```python
from build123d import *

# Parameters (mm, degrees)
BOSS_EXTRUDE1_DEPTH              = 20
CUT_EXTRUDE1_DEPTH               = 80
M14X2_0_TAPPED_HOLE2_D           = 12
M14X2_0_TAPPED_HOLE2_CSINK_D     = 14.05
M14X2_0_TAPPED_HOLE2_CSINK_ANGLE = 90
SKETCH11_W                       = 26
SKETCH11_H                       = 50
BOSS_EXTRUDE2_DEPTH              = 60
BOSS_EXTRUDE3_START              = 4
SKETCH12_R                       = 24.50968872
BOSS_EXTRUDE3_DEPTH              = 34
BOSS_EXTRUDE4_START              = 4
SKETCH13_R                       = 24.725624797
BOSS_EXTRUDE4_DEPTH              = 34
SKETCH14_R                       = 10
CUT_EXTRUDE2_DEPTH               = 234
SKETCH15_W                       = 34
SKETCH15_H                       = 100.230824912
CUT_EXTRUDE3_DEPTH               = 6
RIB6_REACH                       = 189.964
SKETCH16_WALL_W                  = 418.569099694
SKETCH16_WALL_H                  = 16


with BuildPart() as part:
    # Sketch1 → Boss-Extrude1 (new body)
    with BuildSketch(Plane.XY):
        with BuildLine():
            Line((-165.913043478, -4.304347826), (54.086956522, -4.304347826))
            ThreePointArc((54.086956522, -4.304347826), (79.086956522, 20.695652174), (54.086956522, 45.695652174))
            Line((54.086956522, 45.695652174), (-165.913043478, 45.695652174))
            Line((-165.913043478, 45.695652174), (-165.913043478, 28.695652174))
            Line((-165.913043478, 28.695652174), (-149.913043478, 28.695652174))
            ThreePointArc((-149.913043478, 28.695652174), (-141.913043478, 20.695652174), (-149.913043478, 12.695652174))
            Line((-149.913043478, 12.695652174), (-165.913043478, 12.695652174))
            Line((-165.913043478, 12.695652174), (-165.913043478, -4.304347826))
        make_face()
    extrude(amount=BOSS_EXTRUDE1_DEPTH)

    # Sketch2 → Cut-Extrude1 (cut)
    with BuildSketch(Plane(origin=(0, 45.695652174, 0), x_dir=(1, 0, 0), z_dir=(0, 1, 0))):
        with BuildLine():
            Line((-80.413043478, -20), (-6.413043478, -20))
            Line((-6.413043478, -20), (-6.413043478, -18))
            ThreePointArc((-6.413043478, -18), (-7.584616354, -15.171572875), (-10.413043478, -14))
            Line((-10.413043478, -14), (-76.413043478, -14))
            ThreePointArc((-76.413043478, -14), (-79.241470603, -15.171572875), (-80.413043478, -18))
            Line((-80.413043478, -18), (-80.413043478, -20))
        make_face()
    extrude(amount=-CUT_EXTRUDE1_DEPTH, mode=Mode.SUBTRACT)

    # M14x2.0 Tapped Hole2 (through all)
    with Locations(Plane(origin=(0, 0, 0), x_dir=(-1, 0, 0), z_dir=(0, 0, -1))):
        with Locations((-54.086956522, 20.695652174)):
            CounterSinkHole(M14X2_0_TAPPED_HOLE2_D / 2, M14X2_0_TAPPED_HOLE2_CSINK_D / 2, counter_sink_angle=M14X2_0_TAPPED_HOLE2_CSINK_ANGLE)

    # Sketch11 → Boss-Extrude2 (add)
    with BuildSketch(Plane(origin=(0, 0, 0), x_dir=(-1, 0, 0), z_dir=(0, 0, -1))):
        with Locations((97.413043478, 20.695652174)):
            Rectangle(SKETCH11_W, SKETCH11_H)
        with Locations((-10.586956522, 20.695652174)):
            Rectangle(SKETCH11_W, SKETCH11_H)
    extrude(amount=BOSS_EXTRUDE2_DEPTH)

    # Sketch12 → Boss-Extrude3 (add)
    with BuildSketch(Plane.ZY.offset(110.413043478).offset(BOSS_EXTRUDE3_START)):
        with Locations((-60, 20.695652174)):
            Circle(SKETCH12_R)
    extrude(amount=-BOSS_EXTRUDE3_DEPTH)

    # Sketch13 → Boss-Extrude4 (add)
    with BuildSketch(Plane.ZY.offset(2.413043478).offset(BOSS_EXTRUDE4_START)):
        with Locations(Location((-60, 20.695652174, 0), (0, 0, 270))):
            Circle(SKETCH13_R)
    extrude(amount=-BOSS_EXTRUDE4_DEPTH)

    # Sketch14 → Cut-Extrude2 (cut)
    with BuildSketch(Plane(origin=(27.586956522, 0, 0), x_dir=(0, 0, -1), z_dir=(1, 0, 0))):
        with Locations(Location((60, 20.695652174, 0), (0, 0, 90))):
            Circle(SKETCH14_R)
    extrude(amount=-CUT_EXTRUDE2_DEPTH, mode=Mode.SUBTRACT)

    # Sketch15 → Cut-Extrude3 (cut)
    with BuildSketch(Plane(origin=(27.586956522, 0, 0), x_dir=(0, 0, -1), z_dir=(1, 0, 0))):
        with Locations((60, 20.695652174)):
            Rectangle(SKETCH15_W, SKETCH15_H)
    extrude(amount=-CUT_EXTRUDE3_DEPTH, mode=Mode.SUBTRACT)

    # Sketch16 wall → Rib6 (add, up to next)
    with BuildSketch(Plane(origin=(-122.592806802, 20.695652174, -18.5875655), x_dir=(-0.404065346257, 0, 0.914730121924), z_dir=(0.914730121924, 0, 0.404065346257)), mode=Mode.PRIVATE) as rib6_sk1:
        Rectangle(SKETCH16_WALL_W, SKETCH16_WALL_H)
    rib6_tool1 = extrude(rib6_sk1.sketch, amount=RIB6_REACH, mode=Mode.PRIVATE) - part.part
    add(rib6_tool1.solids().sort_by_distance((-122.592806802, 20.695652174, -18.5875655))[0])


solid = part.part
```
Can you work these out from the model? Positions are in its coordinate system, mm. A direction names the side the tool comes from. Give positions to 0.01 mm unless a question says otherwise; leave off trailing zeros. Write each loop counter-clockwise with the first axis right and the second up, starting at its lowest first coordinate (ties: lowest second). Pieces come first, ordered by that corner, then holes. Notation, with made-up numbers: (74.5, 42) - (101.5, 42) arc R16 cw to (101.5, 72) - close; hole circle Ø10 at (-25, 3). An arc over 180 degrees is marked (long way). Write item = value, one per line. Start each with the question number.
1. Thinking about a two-plate mould opening in Z: for faces 1 (the face through (-110.413, 37, -23)), 2 (the face through (-43, 21, 14)), 3 (the face through (-48, -4.304, 1)), which applies, released by +Z, released by -Z, zero draft, split by the parting line, or undercut?
2. Please list where these lines run through material, in increasing order: line 1 (X direction, y = 8.5, z = -35); line 2 (Z direction, x = -83, y = 15.5); line 3 (X direction, y = 29, z = -39).
3. Imagine slicing it at D-D (y = -1). Please give me the cut outline in (x, z).
4. For pin 1 (24 mm diameter, centred on y = 9.5, z = -65.5, fed in from -X); pin 2 (5 mm diameter, centred on x = 24, y = 19.5, fed in from -Z); pin 3 (4 mm diameter, centred on x = -87.5, z = -66.5, fed in from -Y), each with a flat end and sliding along its axis, tell me the tip position at first contact or that it passes through.
5. On a 3-axis mill with a long thin cutter (end or side, diameter ignored), from which of +Z, -Z, +X, -X, +Y, -Y can I reach the whole of each face in a straight line? I mean faces 4 (the face through (21.587, 21, -48)), 5 (the face through (25.559, 20.414, -35.276)), 6 (the face through (-118, 28.696, -12)), 7 (the face through (6.571, 26.056, -84.138)). Say none if no direction works.
6. Imagine slicing it at C-C (y = 23). Count the separate pieces of the cut face and the enclosed holes in it, and give its area (3 significant figures).
7. Imagine slicing it at B-B (z = -6.5). Please give me the cut outline in (x, y).
Worked answers:
q1.face_1 = undercut
q1.face_2 = released by +Z
q1.face_3 = zero draft
q2.line_1 = -110.41 to -84.41, -2.41 to 23.59
q2.line_2 = -83.95 to -68.54, -51.46 to -36.05, 0 to 20
q2.line_3 = -114.41 to -80.41, -6.41 to 27.59
q3.outline = (-165.91, 0) - (-110.41, 0) - (-110.41, -48.6) - (-114.41, -48.6) - (-114.41, -71.4) - (-80.41, -71.4) - (-80.41, -48.6) - (-84.41, -48.6) - (-84.41, 0) - (-2.41, 0) - (-2.41, -48.14) - (-6.41, -48.14) - (-6.41, -71.86) - (21.59, -71.86) - (21.59, -43) - (23.59, -43) - (23.59, 0) - (66.51, 0) - (66.51, 20) - (-6.41, 20) - (-6.41, 18) arc R4 cw to (-10.41, 14) - (-76.41, 14) arc R4 cw to (-80.41, 18) - (-80.41, 20) - (-165.91, 20) - close
q4.pin_1 = -114.41
q4.pin_2 = -84.73
q4.pin_3 = -3.4
q5.face_4 = +X, +Y, -Y
q5.face_5 = +X
q5.face_6 = -X, +Y
q5.face_7 = none
q6.separate_pieces = 4
q6.enclosed_holes = 0
q6.area = 7,980 mm2
q7.outline = (-127.93, 12.7) - (-110.41, 12.7) - (-110.41, -4.3) - (-84.41, -4.3) - (-84.41, 45.7) - (-110.41, 45.7) - (-110.41, 28.7) - (-127.93, 28.7) - close; (-2.41, -4.3) - (23.59, -4.3) - (23.59, 45.7) - (-2.41, 45.7) - close
